For this review, use the dimensioned drawing (mm, ordinates from the lowest corner) and the shaded views. Round coordinates to 2 decimals unless told otherwise and drop trailing zeros. Write each question's results on one line, items separated by ' | '.
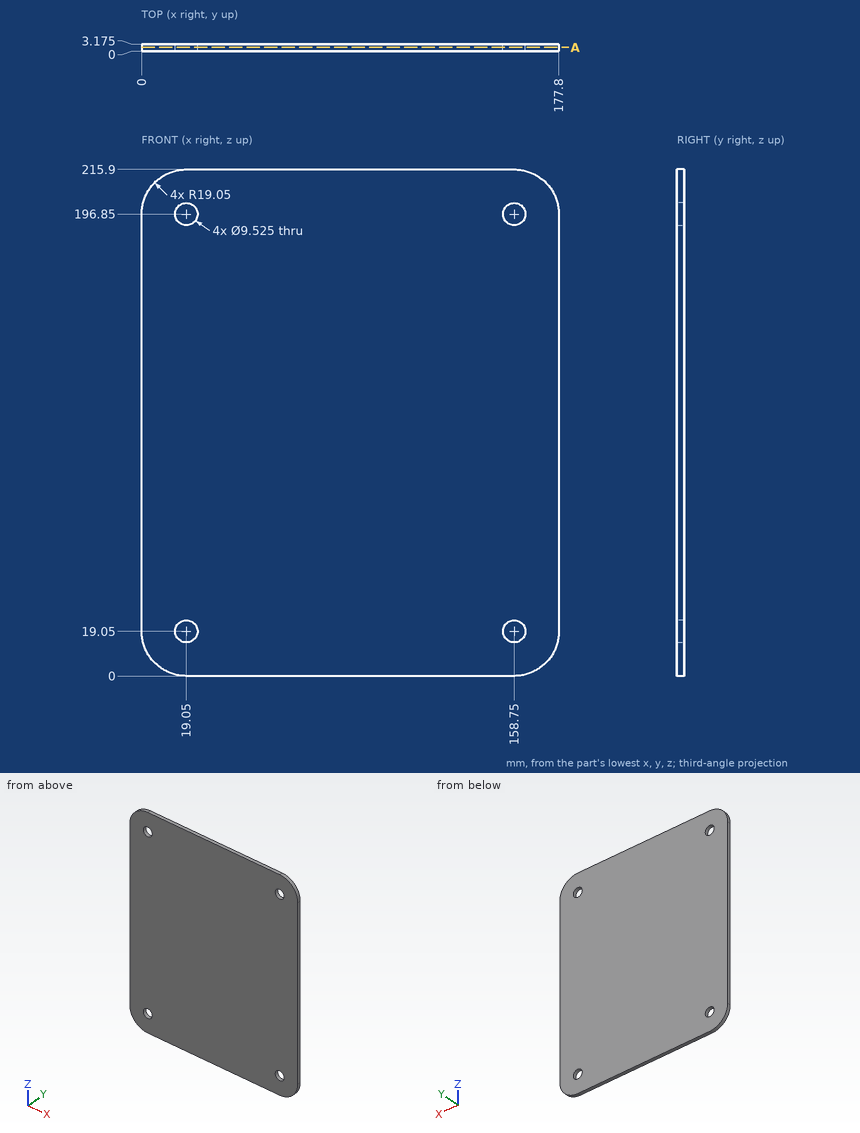
Q1. Insertion check: P1, Ø11, axis at x = 158.75, z = 196.85, coming from the +Y side (3 decimals); P2, Ø7.5, axis at x = 158.75, z = 19.05, coming from the +Y side. Each pin has a flat end and moves straight along its axis. Give the tip position at first contact, or say it passes through.
Evaluation:
P1: stops at y = 3.175 | P2: passes through
Q2. We need section A-A (y = 1.7). State how many separate pieces and enclosed holes the cut face has, plus the area to 3 significant figures.
Evaluation:
separate pieces: 1 | enclosed holes: 4 | area: 37,800 mm^2
Q3. For probe 1 along X at (y, z) = (2.3, 19.05); probe 2 along Z at (x, y) = (158.5, 0.6); probe 3 along Z at (x, y) = (21, 2.35), list the stretches that pass through material, from the lowest coordinate up.
Evaluation:
probe 1: x = 0 to 14.29, 23.81 to 153.99, 163.51 to 177.8 | probe 2: z = 0 to 14.29, 23.81 to 192.09, 201.61 to 215.9 | probe 3: z = 0 to 14.71, 23.39 to 192.51, 201.19 to 215.9
